```python
from build123d import *

# Parameters (mm, degrees)
SKETCH_1_R                  = 1.7
SKETCH_1_R_2                = 2
SKETCH_1_W                  = 20.3
SKETCH_1_H                  = 41.3
F_07_TILT_DRIVE_CHEEK_DEPTH = 6


with BuildPart() as part:
    # Эскиз1 → 07_Tilt_drive_cheek (new body)
    with BuildSketch(Plane.XY):
        Polygon((-38, 0), (38, 0), (38, 62), (22, 88), (-22, 88), (-38, 62), align=None)
        with Locations((-5, 21.75)):
            Circle(SKETCH_1_R, mode=Mode.SUBTRACT)
        with Locations((-5, 71.25)):
            Circle(SKETCH_1_R, mode=Mode.SUBTRACT)
        with Locations((5, 21.75)):
            Circle(SKETCH_1_R, mode=Mode.SUBTRACT)
        with Locations((5, 71.25)):
            Circle(SKETCH_1_R, mode=Mode.SUBTRACT)
        with Locations((-24, 10)):
            Circle(SKETCH_1_R_2, mode=Mode.SUBTRACT)
        with Locations((24, 10)):
            Circle(SKETCH_1_R, mode=Mode.SUBTRACT)
        with Locations((0, 46.5)):
            Rectangle(SKETCH_1_W, SKETCH_1_H, mode=Mode.SUBTRACT)
    extrude(amount=F_07_TILT_DRIVE_CHEEK_DEPTH)


solid = part.part
```
The listing builds one solid part. Answer for the finished solid, in the listing's coordinates (mm). A direction names the side the tool comes from. Coordinates: 2 decimals unless noted, no trailing zeros. Write each loop counter-clockwise with the first axis right and the second up, starting at its lowest first coordinate (ties: lowest second). Pieces come first, ordered by that corner, then holes. Notation, with made-up numbers: (-29.75, 1) - (22.25, 1) arc R26 cw to (22.25, 25) - close; hole circle Ø7 at (20, 30). An arc over 180 degrees is marked (long way). Return JSON: item names as keys, results as strings. Group by question number.
1. A cutting plane is placed at D-D, the plane z = 1.4. Determine the outline of the cut face in (x, y), plus the area to 3 significant figures.
2. Straight lines are drawn through the part: L1, parallel to Y at x = 5, z = 4.55; L2, parallel to X at y = 22, z = 2.05; L3, parallel to X at y = 60, z = 4.3. For each, find the intervals that lie inside material, in ascending order.
3. A cutting plane is placed at B-B, the plane x = -9. Determine the outline of the cut face in (y, z), plus the area to 3 significant figures.
4. A cutting plane is placed at A-A, the plane y = 31. Determine the outline of the cut face in (x, z), plus the area to 3 significant figures.
5. Which of the six approach directions +Z, -Z, +X, -X, +Y, -Y give full straight-line access (tool end or side, diameter ignored) to faces 1 (the flat face through (0, 25.85, 3)), 2 (the flat face through (-1, 0, 3))?
6. A cutting plane is placed at C-C, the plane y = 21.75. Determine the outline of the cut face in (x, z), plus the area to 3 significant figures.
7. Determine the mould class of faces 3 (the flat face through (-1, 25, 6)), 4 (the flat face through (30, 75, 3)), 5 (the flat face through (-38, 31, 3)), 6 (the cylindrical face through (-25.474, 11.352, 2.958)) for opening direction X: released by +X, released by -X, zero draft, split by the parting line, or undercut.
Ans:
{
 "1": {"outline": "(-38, 0) - (38, 0) - (38, 62) - (22, 88) - (-22, 88) - (-38, 62) - close; hole circle Ø4 at (-24, 10); hole (-10.15, 25.85) - (10.15, 25.85) - (10.15, 67.15) - (-10.15, 67.15) - close; hole circle Ø3.4 at (-5, 21.75); hole circle Ø3.4 at (-5, 71.25); hole circle Ø3.4 at (5, 21.75); hole circle Ø3.4 at (5, 71.25); hole circle Ø3.4 at (24, 10)", "area": "5,380 mm²"},
 "2": {"L1": "0 to 20.05, 23.45 to 25.85, 67.15 to 69.55, 72.95 to 88", "L2": "-38 to -6.68, -3.32 to 3.32, 6.68 to 38", "L3": "-38 to -10.15, 10.15 to 38"},
 "3": {"outline": "(0, 0) - (25.85, 0) - (25.85, 6) - (0, 6) - close; (67.15, 0) - (88, 0) - (88, 6) - (67.15, 6) - close", "area": "280 mm²"},
 "4": {"outline": "(-38, 0) - (-10.15, 0) - (-10.15, 6) - (-38, 6) - close; (10.15, 0) - (38, 0) - (38, 6) - (10.15, 6) - close", "area": "334 mm²"},
 "5": {"face 1": "+Z, -Z", "face 2": "+Z, -Z, +X, -X, -Y"},
 "6": {"outline": "(-38, 0) - (-6.7, 0) - (-6.7, 6) - (-38, 6) - close; (-3.3, 0) - (3.3, 0) - (3.3, 6) - (-3.3, 6) - close; (6.7, 0) - (38, 0) - (38, 6) - (6.7, 6) - close", "area": "415 mm²"},
 "7": {"face 3": "zero draft", "face 4": "released by +X", "face 5": "released by -X", "face 6": "undercut"}
}
